The model under review builds one solid part; all positions refer to its coordinate system, in mm. A direction names the side the tool comes from. Give positions to 0.01 mm unless a question says otherwise; leave off trailing zeros. Loops run counter-clockwise (first coordinate to the right, second up) from the corner with the lowest first, then second, coordinate; pieces in that order, holes last. Notation, with made-up numbers: (87.5, -31.75) - (95.5, -31.75) arc R32 cw to (95.5, -0.75) - close; hole circle Ø10 at (-30, 64.25). An arc over 180 degrees is marked (long way). Answer as a JSON object with one key per item and string values.
from build123d import *

# Parameters (mm, degrees)
SMUSSO1_SIZE             = 3
SCHIZZO2_R               = 18.679375542
SCHIZZO2_W               = 20
SCHIZZO2_H               = 20
TAGLIO_ESTRUSIONE1_DEPTH = 17.9
SCHIZZO3_W               = 20
SCHIZZO3_H               = 20
TAGLIO_ESTRUSIONE2_DEPTH = 2.5
SMUSSO2_SIZE             = 1


with BuildPart() as part:
    # Schizzo1 → Rivoluzione1 (revolve)
    with BuildSketch(Plane.XY, mode=Mode.PRIVATE) as rivoluzione1_sk:
        Polygon((8.15, -4.65), (8.15, 10.95), (14, 10.95), (14, 6.95), (10.8, 6.95), (10.8, -5.05), (9.85, -5.05), (9.85, -10.95), (5.1, -10.95), (5.1, -4.65), align=None)
    revolve(rivoluzione1_sk.sketch.rotate(Axis((0, 15.297202797, 0), (0, -1, 0)), 90), axis=Axis((0, 15.297202797, 0), (0, -1, 0)))

    # Smusso1
    smusso1_edges = [part.edges().sort_by_distance(p)[0] for p in [
        (0, 10.95, -14),
    ]]
    chamfer(smusso1_edges, length=SMUSSO1_SIZE)

    # Schizzo2 → Taglio-Estrusione1 (cut)
    with BuildSketch(Plane.XZ.offset(10.95)):
        Circle(SCHIZZO2_R)
        Rectangle(SCHIZZO2_W, SCHIZZO2_H, mode=Mode.SUBTRACT)
    extrude(amount=-TAGLIO_ESTRUSIONE1_DEPTH, mode=Mode.SUBTRACT)

    # Schizzo3 → Taglio-Estrusione2 (cut)
    with BuildSketch(Plane.XZ.offset(10.95)):
        with Locations((7.05, 7.05)):
            Rectangle(SCHIZZO3_W, SCHIZZO3_H)
    extrude(amount=-TAGLIO_ESTRUSIONE2_DEPTH, mode=Mode.SUBTRACT)

    # Smusso2
    smusso2_edges = [part.edges().sort_by_distance(p)[0] for p in [
        (-6.965001795, -10.95, -6.965001795),
    ]]
    chamfer(smusso2_edges, length=SMUSSO2_SIZE)


solid = part.part
Q1. Clearance check with flat-ended pins moving along their axes: pin 1 Ø2 at (x, y) = (8, -9.5) entering from +Z; pin 2 Ø2.5 at (y, z) = (2.5, 0.5) entering from -X; pin 3 Ø6 at (x, y) = (8, -1.5) entering from +Z. State where each tip first meets the part, or that it passes through.
Results:
{"pin 1": "stops at z = -2.95", "pin 2": "stops at x = -10", "pin 3": "stops at z = 9.57"}
Q2. For faces 1 (the face through (10, 1, 0)), 2 (the face through (-2.95, -10, 7)), 3 (the face through (7.594, 0.866, -7.679)), 4 (the face through (-10, 1, 0)), list the 3-axis set-ups (+Z, -Z, +X, -X, +Y, -Y) from which the entire face can be reached by the end or side of a thin tool; tool diameter is ignored.
Results:
{"face 1": "+Z, -Z, +X, -Y", "face 2": "+Z, +X, -Y", "face 3": "-Z, +X, -Y", "face 4": "+Z, -Z, -X, -Y"}
Q3. To check wall thickness, follow probe 1 along X at (y, z) = (3.75, 0); probe 2 along Z at (x, y) = (4.5, 7.5); probe 3 along X at (y, z) = (4.5, 1.5). State the ranges of each line that lie inside material, in increasing order. Write a range as [from, to].
Results:
{"probe 1": "x = [-10, -8.15], [8.15, 10]", "probe 2": "z = [-13.26, -6.8], [6.8, 13.26]", "probe 3": "x = [-10, -8.01], [8.01, 10]"}
Q4. The part is to be moulded in two halves that separate along Z. For faces 5 (the face through (7, -10, -2.95)), 6 (the face through (4.959, 3.259, -6.468)), 7 (the face through (-1.1, 6.95, 10.3)), say which applies: +Z half, -Z half, draft (parallel to the pull), parting line (faces both ways), or undercut.
Results:
{"face 5": "+Z half", "face 6": "undercut", "face 7": "draft"}
Q5. Consider section A-A, the plane y = 0.25. State the section outline as (x, z) points, plus the area to 3 significant figures.
Results:
{"outline": "(-10, -4.08) arc R10.8 ccw to (-4.08, -10) - (4.08, -10) arc R10.8 ccw to (10, -4.08) - (10, 4.08) arc R10.8 ccw to (4.08, 10) - (-4.08, 10) arc R10.8 ccw to (-10, 4.08) - close; hole circle Ø16.3 at (0, 0)", "area": "140 mm^2"}
Q6. Consider section B-B, the plane z = 0. State the section outline as (x, y) points, plus the area to 3 significant figures.
Results:
{"outline": "(-14, 6.95) - (-10, 6.95) - (-10, -5.05) - (-9.85, -5.05) - (-9.85, -9.95) - (-8.85, -10.95) - (-5.1, -10.95) - (-5.1, -4.65) - (-8.15, -4.65) - (-8.15, 10.95) - (-11, 10.95) - (-14, 7.95) - close; (5.1, -8.45) - (9.85, -8.45) - (9.85, -5.05) - (10, -5.05) - (10, 6.95) - (14, 6.95) - (14, 7.95) - (11, 10.95) - (8.15, 10.95) - (8.15, -4.65) - (5.1, -4.65) - close", "area": "128 mm^2"}
Q7. Consider section D-D, the plane y = -7.5. State the section outline as (x, z) points, plus the area to 3 significant figures.
Results:
{"outline": "circle Ø19.7 at (0, 0); hole circle Ø10.2 at (0, 0)", "area": "223 mm^2"}
Q8. Consider section C-C, the plane x = 0. State the section outline as (y, z) points.
Results:
{"outline": "(-10.95, -8.85) - (-9.95, -9.85) - (-5.05, -9.85) - (-5.05, -10) - (6.95, -10) - (6.95, -14) - (7.95, -14) - (10.95, -11) - (10.95, -8.15) - (-4.65, -8.15) - (-4.65, -5.1) - (-10.95, -5.1) - close; (-8.45, 5.1) - (-4.65, 5.1) - (-4.65, 8.15) - (10.95, 8.15) - (10.95, 11) - (7.95, 14) - (6.95, 14) - (6.95, 10) - (-5.05, 10) - (-5.05, 9.85) - (-8.45, 9.85) - close"}
